Could you check a few things on this model? Use its own coordinates, in mm. A direction names the side the tool comes from. Give positions to 0.01 mm unless a question says otherwise; leave off trailing zeros. Write each loop counter-clockwise with the first axis right and the second up, starting at its lowest first coordinate (ties: lowest second). Pieces come first, ordered by that corner, then holes. Notation, with made-up numbers: (-5, 27) - (52, 27) arc R13 ccw to (52, 41) - close; hole circle Ø10 at (-21, 37). An arc over 180 degrees is marked (long way). Use one line per item in the form item = value.
```python
from build123d import *

# Parameters (mm, degrees)
SKETCH1_W           = 76.2
SKETCH1_H           = 177.8
BOSS_EXTRUDE1_DEPTH = 3.175
SKETCH2_R           = 1.3843
SKETCH2_W           = 50.8
SKETCH2_H           = 152.4
CUT_EXTRUDE1_DEPTH  = 182.864044344


with BuildPart() as part:
    # Sketch1 → Boss-Extrude1 (new body)
    with BuildSketch(Plane(origin=(0, 0, 0), x_dir=(1, 0, 0), z_dir=(0, 1, 0))):
        with Locations((0, -88.9)):
            Rectangle(SKETCH1_W, SKETCH1_H)
    extrude(amount=BOSS_EXTRUDE1_DEPTH)

    # Sketch2 → Cut-Extrude1 (cut, through all)
    with BuildSketch(Plane(origin=(0, 3.175, 0), x_dir=(1, 0, 0), z_dir=(0, 1, 0))):
        with Locations(Location((0, -6.35, 0), (0, 0, 270))):
            Circle(SKETCH2_R)
        with Locations(Location((0, -171.45, 0), (0, 0, 270))):
            Circle(SKETCH2_R)
        with Locations(Location((-28.8671, -13.1191, 0), (0, 0, 270))):
            Circle(SKETCH2_R)
        with Locations(Location((28.8671, -13.1191, 0), (0, 0, 270))):
            Circle(SKETCH2_R)
        with Locations(Location((-28.8671, -164.6809, 0), (0, 0, 270))):
            Circle(SKETCH2_R)
        with Locations(Location((28.8671, -164.6809, 0), (0, 0, 270))):
            Circle(SKETCH2_R)
        with Locations((0, -88.9)):
            Rectangle(SKETCH2_W, SKETCH2_H)
    extrude(amount=-CUT_EXTRUDE1_DEPTH, mode=Mode.SUBTRACT)


solid = part.part
```
1. Imagine slicing it at A-A, the plane z = 39. List the corners of the cut face in (x, y) for me (3 decimals), and give its area (3 significant figures).
Response values:
outline = (-38.1, 0) - (-25.4, 0) - (-25.4, 3.175) - (-38.1, 3.175) - close; (25.4, 0) - (38.1, 0) - (38.1, 3.175) - (25.4, 3.175) - close
area = 80.6 mm²
2. Which directions (+Z, -Z, +X, -X, +Y, -Y) give clear straight access to the entire face, cutting with the end or side of a thin tool? Please do faces 1 (the face through (-25.4, 2, 90)), 2 (the face through (38.1, 2, 90)).
Response values:
face_1 = +Y, -Y
face_2 = +Z, -Z, +X, +Y, -Y
3. Imagine slicing it at B-B, the plane x = 19.5. List the corners of the cut face in (y, z) for me (3 decimals).
Response values:
outline = (0, 0) - (3.175, 0) - (3.175, 12.7) - (0, 12.7) - close; (0, 165.1) - (3.175, 165.1) - (3.175, 177.8) - (0, 177.8) - close
4. If I drill on line 1 (X direction, y = 1.45, z = 111); line 2 (Z direction, x = -20, y = 2.75); line 3 (Z direction, x = -28.5, y = 0.6), over which ranges is the centre line in solid material (lowest first)? Write a range as from..to.
Response values:
line_1 = -38.1..-25.4, 25.4..38.1
line_2 = 0..12.7, 165.1..177.8
line_3 = 0..11.78, 14.45..163.35, 166.02..177.8
5. If we mould it in two halves opening along X, with no side actions, what happens to faces 3 (the face through (-26, 0, 88)), 4 (the face through (-38.1, 2, 90)), 5 (the face through (0, 2, 12.7))? For each: pulls with the +X half, pulls with the -X half, needs draft (parallel to the pull), parting line crosses it, or undercut.
Response values:
face_3 = needs draft
face_4 = pulls with the -X half
face_5 = undercut
6. For pin 1 (2.5 mm diameter, centred on x = 0, z = 171.45, fed in from +Y); pin 2 (4.5 mm diameter, centred on x = 28.87, z = 13.12, fed in from +Y) (3 decimals), each with a flat end and sliding along its axis, tell me the tip position at first contact or that it passes through.
Response values:
pin_1 = through
pin_2 = 3.175
